Here's the drawing with two shaded views (mm, measured from the low corner). I have some questions. Coordinates: 2 decimals unless noted, no trailing zeros. Loops run counter-clockwise (first coordinate to the right, second up) from the corner with the lowest first, then second, coordinate; pieces in that order, holes last. Notation, with made-up numbers: (49, 37.5) - (53, 37.5) arc R28 cw to (53, 69.5) - close; hole circle Ø1 at (55.25, 36.5). An arc over 180 degrees is marked (long way). Use a Markdown table: item, result.
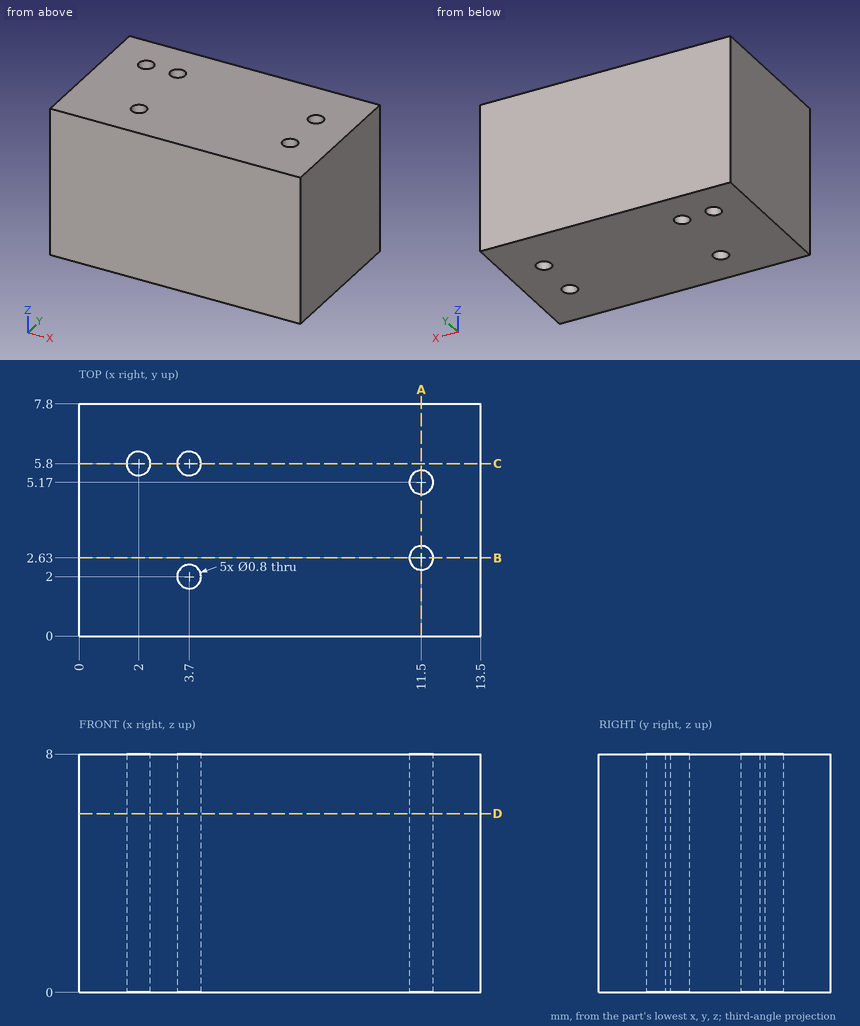
Q1. I want a section at C-C, the plane y = 5.8. Write out the boundary of the cut face in (x, z), then the cut area to 3 significant figures.
Check values:
| item | result |
|---|---|
| outline | (0, 0) - (1.6, 0) - (1.6, 8) - (0, 8) - close; (2.4, 0) - (3.3, 0) - (3.3, 8) - (2.4, 8) - close; (4.1, 0) - (13.5, 0) - (13.5, 8) - (4.1, 8) - close |
| area | 95.2 mm^2 |
Q2. I want a section at D-D, the plane z = 6. Write out the boundary of the cut face in (x, y).
Check values:
| item | result |
|---|---|
| outline | (0, 0) - (13.5, 0) - (13.5, 7.8) - (0, 7.8) - close; hole circle Ø0.8 at (2, 5.8); hole circle Ø0.8 at (3.7, 2); hole circle Ø0.8 at (3.7, 5.8); hole circle Ø0.8 at (11.5, 2.63); hole circle Ø0.8 at (11.5, 5.17) |
Q3. I want a section at B-B, the plane y = 2.63. Write out the boundary of the cut face in (x, z).
Check values:
| item | result |
|---|---|
| outline | (0, 0) - (11.1, 0) - (11.1, 8) - (0, 8) - close; (11.9, 0) - (13.5, 0) - (13.5, 8) - (11.9, 8) - close |
Q4. I want a section at A-A, the plane x = 11.5. Write out the boundary of the cut face in (y, z).
Check values:
| item | result |
|---|---|
| outline | (0, 0) - (2.23, 0) - (2.23, 8) - (0, 8) - close; (3.03, 0) - (4.77, 0) - (4.77, 8) - (3.03, 8) - close; (5.57, 0) - (7.8, 0) - (7.8, 8) - (5.57, 8) - close |
Q5. Please list where these lines run through material, in increasing order: L1, parallel to Y at x = 11.5, z = 6; L2, parallel to X at y = 5.75, z = 6; L3, parallel to Y at x = 2, z = 3. Write a range as from..to.
Check values:
| item | result |
|---|---|
| L1 | 0..2.23, 3.03..4.77, 5.57..7.8 |
| L2 | 0..1.6, 2.4..3.3, 4.1..13.5 |
| L3 | 0..5.4, 6.2..7.8 |
